Could you check a few things on this drawing? It's one solid part, dimensions in mm from its lowest x, y, z. A direction names the side the tool comes from. Give positions to 0.01 mm unless a question says otherwise; leave off trailing zeros. Order: outer loops, then holes, each group sorted by start corner. A loop starts at its lowest first (then second) coordinate and runs counter-clockwise, first axis right, second up. Notation, with made-up numbers: (65.5, -25.75) - (103.5, -25.75) arc R18 ccw to (103.5, -19.75) - close; hole circle Ø10 at (34, 27.5). An arc over 180 degrees is marked (long way). Answer as CSV lines item,"result".
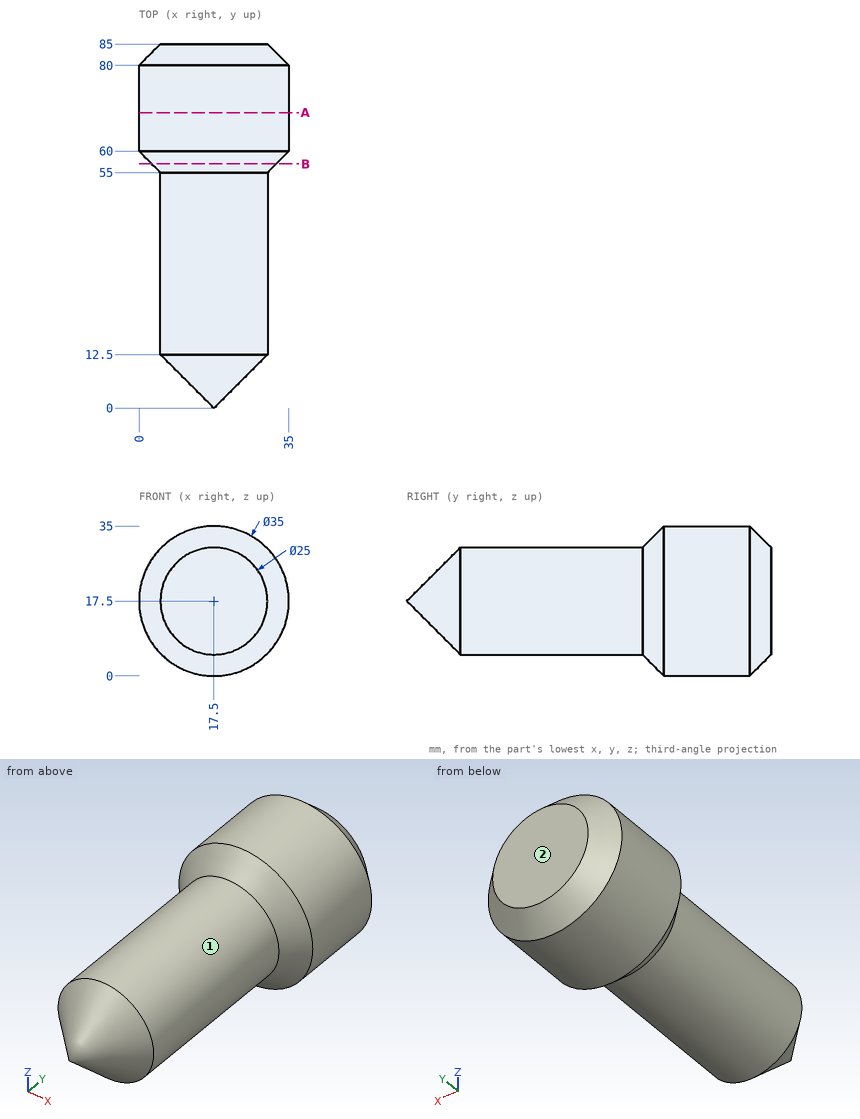
1) I need wall thicknesses on line 1 along Z through (x, y) = (4, 59.5); line 2 along Z through (x, y) = (6, 75); line 3 along Y through (x, z) = (14, 8.5). Which ranges of each line are inside material? Lowest first, please. Write a range as [from, to].
Answer block:
line 1,"[7.17, 27.83]"
line 2,"[4.31, 30.69]"
line 3,"[9.66, 85]"
2) I want a section at A-A on y = 69. Write out the boundary of the cut face in (x, z).
Answer block:
outline,"circle Ø35 at (17.5, 17.5)"
3) I want a section at B-B on y = 57. Write out the boundary of the cut face in (x, z).
Answer block:
outline,"circle Ø29 at (17.5, 17.5)"
4) Which directions (+Z, -Z, +X, -X, +Y, -Y) give clear straight access to the entire face, cutting with the end or side of a thin tool? Please do the marked faces 1 and 2.
Answer block:
face 1,"-Y"
face 2,"+Z, -Z, +X, -X, +Y"
5) I'm going to push flat-ended pins straight in: P1, Ø3, axis at x = 15, y = 74, coming from the +Z side; P2, Ø6, axis at x = 20.5, y = 29, coming from the -Z side; P3, Ø12, axis at x = 5.5, y = 29.5, coming from the +Z side. Where does each tip first touch, or does it pass through?
Answer block:
P1,"z = 34.97"
P2,"z = 5"
P3,"z = 28.47"
